from build123d import *

# Parameters (mm, degrees)
SKETCH1_W           = 100
SKETCH1_H           = 100
BOSS_EXTRUDE1_DEPTH = 5
SKETCH2_W           = 10
SKETCH2_H           = 30
BOSS_EXTRUDE2_DEPTH = 50
CUT_EXTRUDE2_DEPTH  = 6
FILLET1_R           = 5
FILLET2_R           = 5
SKETCH7_W           = 0.707106782
SKETCH7_H           = 0.707106782
CUT_EXTRUDE3_DEPTH  = 1.5
SKETCH10_R          = 2.4
CUT_EXTRUDE4_DEPTH  = 11
CHAMFER1_SIZE       = 0.5
CHAMFER2_SIZE       = 0.5
CHAMFER3_SIZE       = 0.5
SKETCH11_W          = 1
SKETCH11_H          = 1
BOSS_EXTRUDE3_DEPTH = 2.5


with BuildPart() as part:
    # Sketch1 → Boss-Extrude1 (new body)
    with BuildSketch(Plane(origin=(0, 0, 0), x_dir=(1, 0, 0), z_dir=(0, 1, 0))):
        Rectangle(SKETCH1_W, SKETCH1_H)
    extrude(amount=BOSS_EXTRUDE1_DEPTH)

    # Sketch2 → Boss-Extrude2 (add)
    with BuildSketch(Plane(origin=(0, 5, 0), x_dir=(1, 0, 0), z_dir=(0, 1, 0))):
        with Locations((-45, 5.85)):
            Rectangle(SKETCH2_W, SKETCH2_H)
        with Locations((45, 0)):
            Rectangle(SKETCH2_W, SKETCH2_H)
    extrude(amount=BOSS_EXTRUDE2_DEPTH)

    # Sketch4 → Cut-Extrude2 (cut, through all)
    with BuildSketch(Plane(origin=(0, 5, 0), x_dir=(1, 0, 0), z_dir=(0, 1, 0))):
        with BuildLine():
            Line((-1.91, -1.46), (1.91, -1.46))
            ThreePointArc((1.91, -1.46), (2.263553391, -1.313553391), (2.41, -0.96))
            Line((2.41, -0.96), (2.41, 0.96))
            ThreePointArc((2.41, 0.96), (2.263553391, 1.313553391), (1.91, 1.46))
            Line((1.91, 1.46), (-1.91, 1.46))
            ThreePointArc((-1.91, 1.46), (-2.263553391, 1.313553391), (-2.41, 0.96))
            Line((-2.41, 0.96), (-2.41, -0.96))
            ThreePointArc((-2.41, -0.96), (-2.263553391, -1.313553391), (-1.91, -1.46))
        make_face()
    extrude(amount=-CUT_EXTRUDE2_DEPTH, mode=Mode.SUBTRACT)

    # Fillet1
    fillet1_edges = [part.edges().sort_by_distance(p)[0] for p in [
        (50, 2.5, 50),
        (-50, 2.5, 50),
        (-50, 2.5, -50),
        (50, 2.5, -50),
    ]]
    fillet(fillet1_edges, radius=FILLET1_R)

    # Fillet2
    fillet2_edges = [part.edges().sort_by_distance(p)[0] for p in [
        (-45, 55, 9.15),
        (-45, 55, -20.85),
        (45, 55, -15),
        (45, 55, 15),
    ]]
    fillet(fillet2_edges, radius=FILLET2_R)

    # Sketch7 → Cut-Extrude3 (cut)
    with BuildSketch(Plane(origin=(-40, 0, 0), x_dir=(0, 0, -1), z_dir=(1, 0, 0))):
        with BuildLine():
            Line((7.65, 31.7), (7.65, 37.11555898))
            ThreePointArc((7.65, 37.11555898), (8.211651546, 37.554064192), (8.669574436, 38.1))
            Line((8.669574436, 38.1), (14.05, 38.1))
            ThreePointArc((14.05, 38.1), (15.95, 40), (14.05, 41.9))
            Line((14.05, 41.9), (8.669574436, 41.9))
            ThreePointArc((8.669574436, 41.9), (8.211651546, 42.445935808), (7.65, 42.88444102))
            Line((7.65, 42.88444102), (7.65, 48.3))
            ThreePointArc((7.65, 48.3), (5.85, 50.1), (4.05, 48.3))
            Line((4.05, 48.3), (4.05, 42.88444102))
            ThreePointArc((4.05, 42.88444102), (3.488348454, 42.445935808), (3.030425564, 41.9))
            Line((3.030425564, 41.9), (-2.35, 41.9))
            ThreePointArc((-2.35, 41.9), (-4.25, 40), (-2.35, 38.1))
            Line((-2.35, 38.1), (3.030425564, 38.1))
            ThreePointArc((3.030425564, 38.1), (3.488348454, 37.554064192), (4.05, 37.11555898))
            Line((4.05, 37.11555898), (4.05, 31.7))
            ThreePointArc((4.05, 31.7), (5.85, 29.9), (7.65, 31.7))
        make_face()
        with Locations((-0.45, 40)):
            Rectangle(SKETCH7_W, SKETCH7_H, mode=Mode.SUBTRACT)
        with Locations((5.85, 33.7)):
            Rectangle(SKETCH7_W, SKETCH7_H, mode=Mode.SUBTRACT)
        with Locations((12.15, 40)):
            Rectangle(SKETCH7_W, SKETCH7_H, mode=Mode.SUBTRACT)
        with Locations((5.85, 46.3)):
            Rectangle(SKETCH7_W, SKETCH7_H, mode=Mode.SUBTRACT)
    extrude(amount=-CUT_EXTRUDE3_DEPTH, mode=Mode.SUBTRACT)

    # Sketch10 → Cut-Extrude4 (cut, through all)
    with BuildSketch(Plane.ZY.offset(-40)):
        with Locations((0, 45)):
            Circle(SKETCH10_R)
    extrude(amount=-CUT_EXTRUDE4_DEPTH, mode=Mode.SUBTRACT)

    # Chamfer1
    chamfer1_edges = [part.edges().sort_by_distance(p)[0] for p in [
        (2.263553391, 0, 1.313553391),
        (0, 0, 1.46),
        (-2.263553391, 0, 1.313553391),
        (-2.41, 0, 0),
        (-2.263553391, 0, -1.313553391),
        (0, 0, -1.46),
        (2.263553391, 0, -1.313553391),
        (2.41, 0, 0),
    ]]
    chamfer(chamfer1_edges, length=CHAMFER1_SIZE)

    # Chamfer2
    chamfer2_edges = [part.edges().sort_by_distance(p)[0] for p in [
        (-40, 45.59222051, -4.05),
        (-40, 41.9, -11.359787218),
        (-40, 34.40777949, -4.05),
        (-40, 41.9, -0.340212782),
        (-40, 40, 4.25),
        (-40, 38.1, -0.340212782),
        (-40, 29.9, -5.85),
        (-40, 34.40777949, -7.65),
        (-40, 38.1, -11.359787218),
        (-40, 40, -15.95),
        (-40, 45.59222051, -7.65),
        (-40, 50.1, -5.85),
    ]]
    chamfer(chamfer2_edges, length=CHAMFER2_SIZE)

    # Chamfer3
    chamfer3_edges = [part.edges().sort_by_distance(p)[0] for p in [
        (50, 45, -2.4),
    ]]
    chamfer(chamfer3_edges, length=CHAMFER3_SIZE)

    # Sketch11 → Boss-Extrude3 (add)
    with BuildSketch(Plane(origin=(-40, 0, 0), x_dir=(0, 0, -1), z_dir=(1, 0, 0))):
        with Locations((2.95, 46.3)):
            Rectangle(SKETCH11_W, SKETCH11_H)
        with Locations((8.75, 46.3)):
            Rectangle(SKETCH11_W, SKETCH11_H)
        with Locations((12.15, 43)):
            Rectangle(SKETCH11_W, SKETCH11_H)
        with Locations((12.15, 37)):
            Rectangle(SKETCH11_W, SKETCH11_H)
        with Locations((8.75, 33.7)):
            Rectangle(SKETCH11_W, SKETCH11_H)
        with Locations((2.95, 33.7)):
            Rectangle(SKETCH11_W, SKETCH11_H)
        with Locations((-0.45, 37)):
            Rectangle(SKETCH11_W, SKETCH11_H)
        with Locations((-0.45, 43)):
            Rectangle(SKETCH11_W, SKETCH11_H)
    extrude(amount=BOSS_EXTRUDE3_DEPTH)


solid = part.part
Source: CAD feature listing. Evaluate the final solid. Frame: model axes, mm. A direction names the side the tool comes from. Round coordinates to 2 decimals unless told otherwise and drop trailing zeros. Loops run counter-clockwise (first coordinate to the right, second up) from the corner with the lowest first, then second, coordinate; pieces in that order, holes last.
Q1. Section A-A, the plane y = 16.5. Return loops of the section in (x, z).
Q2. Mould query, pull axis Z, two halves, no side actions, for faces 4 (the face through (48, 3, 49)), 5 (the face through (0, 3, 1.46)), 6 (the face through (-49, 3, -48)). Classes: pulls with the +Z half, pulls with the -Z half, needs draft (parallel to the pull), parting line crosses it, or undercut.
Q3. Ray query, line 1 (X direction, y = 48, z = 6.5); line 2 (Y direction, x = 43, z = 0); line 3 (Y direction, x = -32, z = -38). Return the intervals inside material, ascending.
Q4. Access query for faces 1 (the face through (-45, 27, -20.85)), 2 (the face through (44.684, 42.657, -0.52)), 3 (the face through (-45, 27, 9.15)). Directions: +Z, -Z, +X, -X, +Y, -Y. A direction counts if a zero-diameter tool reaches every point of the face in a straight line with its end or side. Return the directions, or none.
Q5. Section C-C, the plane z = 36. Return loops of the section in (x, y), plus the area to 3 significant figures.
Q6. Section B-B, the plane x = -17. Return loops of the section in (y, z), plus the area to 3 significant figures.
Q7. First-contact query: P1, Ø0.5, axis at x = -38.5, y = 33.5, coming from the -Z side; P2, Ø0.5, axis at x = -41, y = 34, coming from the +Z side; P3, Ø8, axis at x = 46.5, y = 28.5, coming from the +Z side. Flat tips, straight axial feed; report the tip coordinate or a pass-through.
Solutions:
1. outline: (-50, -20.85) - (-40, -20.85) - (-40, 9.15) - (-50, 9.15) - close; (40, -15) - (50, -15) - (50, 15) - (40, 15) - close
2. face 4: pulls with the +Z half
2. face 5: undercut
2. face 6: pulls with the -Z half
3. line 1: x = -50 to -40, 40 to 50
3. line 2: y = 0 to 42.6, 47.4 to 55
3. line 3: y = 0 to 5
4. face 1: -Z, +X, -X, +Y
4. face 2: +X
4. face 3: +Z, -X, +Y
5. outline: (-50, 0) - (50, 0) - (50, 5) - (-50, 5) - close
5. area: 500 mm2
6. outline: (0, -50) - (5, -50) - (5, 50) - (0, 50) - close
6. area: 500 mm2
7. P1: stops at z = -9.25
7. P2: stops at z = 9.15
7. P3: stops at z = 15
